from build123d import *

# Parameters (mm, degrees)
ESQUISSE1_W             = 106
ESQUISSE1_H             = 68
BOSS_EXTRU_1_DEPTH      = 8
ESQUISSE2_R             = 3
BOSS_EXTRU_2_DEPTH      = 4.5
ESQUISSE3_R             = 1.25
ENL_V_MAT_EXTRU_1_DEPTH = 7
ESQUISSE4_W             = 106
ESQUISSE4_H             = 1.5
ENL_V_MAT_EXTRU_3_DEPTH = 65
ESQUISSE10_W            = 96
ESQUISSE10_H            = 58.390488624
ENL_V_MAT_EXTRU_5_DEPTH = 1


with BuildPart() as part:
    # Esquisse1 → Boss.-Extru.1 (new body)
    with BuildSketch(Plane(origin=(0, 0, 0), x_dir=(1, 0, 0), z_dir=(0, 1, 0))):
        Rectangle(ESQUISSE1_W, ESQUISSE1_H)
    extrude(amount=BOSS_EXTRU_1_DEPTH)

    # Esquisse2 → Boss.-Extru.2 (add)
    with BuildSketch(Plane.XZ):
        with Locations(Location((-49.5, 31, 0), (0, 0, 90))):
            Circle(ESQUISSE2_R)
        with Locations(Location((-49.5, -31, 0), (0, 0, 90))):
            Circle(ESQUISSE2_R)
        with Locations(Location((49.5, -31, 0), (0, 0, 270))):
            Circle(ESQUISSE2_R)
        with Locations(Location((49.5, 31, 0), (0, 0, 90))):
            Circle(ESQUISSE2_R)
        with Locations(Location((-30.5, 24.5, 0), (0, 0, 90))):
            Circle(ESQUISSE2_R)
        with Locations(Location((27.5, 24.5, 0), (0, 0, 90))):
            Circle(ESQUISSE2_R)
        with Locations(Location((27.5, -24.5, 0), (0, 0, 90))):
            Circle(ESQUISSE2_R)
        with Locations(Location((-30.5, -24.5, 0), (0, 0, 90))):
            Circle(ESQUISSE2_R)
    extrude(amount=BOSS_EXTRU_2_DEPTH)

    # Esquisse3 → Enlèv. mat.-Extru.1 (cut)
    with BuildSketch(Plane.XZ.offset(4.5)):
        with Locations(Location((-49.5, 31, 0), (0, 0, 270))):
            Circle(ESQUISSE3_R)
        with Locations(Location((49.5, 31, 0), (0, 0, 90))):
            Circle(ESQUISSE3_R)
        with Locations(Location((49.5, -31, 0), (0, 0, 270))):
            Circle(ESQUISSE3_R)
        with Locations(Location((-49.5, -31, 0), (0, 0, 90))):
            Circle(ESQUISSE3_R)
        with Locations(Location((-30.5, 24.5, 0), (0, 0, 270))):
            Circle(ESQUISSE3_R)
        with Locations(Location((27.5, 24.5, 0), (0, 0, 90))):
            Circle(ESQUISSE3_R)
        with Locations(Location((27.5, -24.5, 0), (0, 0, 270))):
            Circle(ESQUISSE3_R)
        with Locations(Location((-30.5, -24.5, 0), (0, 0, 90))):
            Circle(ESQUISSE3_R)
    extrude(amount=-ENL_V_MAT_EXTRU_1_DEPTH, mode=Mode.SUBTRACT)

    # Esquisse4 → Enlèv. mat.-Extru.3 (cut)
    with BuildSketch(Plane(origin=(0, 0, -34), x_dir=(-1, 0, 0), z_dir=(0, 0, -1))):
        with Locations((0, 1.75)):
            Rectangle(ESQUISSE4_W, ESQUISSE4_H)
    extrude(amount=-ENL_V_MAT_EXTRU_3_DEPTH, mode=Mode.SUBTRACT)

    # Esquisse10 → Enlèv. mat.-Extru.5 (cut)
    with BuildSketch(Plane(origin=(0, 8, 0), x_dir=(1, 0, 0), z_dir=(0, 1, 0))):
        Rectangle(ESQUISSE10_W, ESQUISSE10_H)
    extrude(amount=-ENL_V_MAT_EXTRU_5_DEPTH, mode=Mode.SUBTRACT)


solid = part.part
Can you work these out from the model? Positions are in its coordinate system, mm. A direction names the side the tool comes from. Coordinates: 2 decimals unless noted, no trailing zeros. Write each loop counter-clockwise with the first axis right and the second up, starting at its lowest first coordinate (ties: lowest second). Pieces come first, ordered by that corner, then holes.
Q1. Imagine slicing it at C-C, the plane z = 11. List the corners of the cut face in (x, y) for me.
Results found:
outline: (-53, 0) - (53, 0) - (53, 1) - (-53, 1) - close; (-53, 2.5) - (53, 2.5) - (53, 8) - (48, 8) - (48, 7) - (-48, 7) - (-48, 8) - (-53, 8) - close
Q2. Please list where these lines run through material, in increasing order: L1, parallel to X at y = -1.25, z = 31; L2, parallel to X at y = -0.3, z = -24.5; L3, parallel to Y at x = 9, z = 9.5.
Results found:
L1: x = -52.5 to -50.75, -48.25 to -46.5, 46.5 to 48.25, 50.75 to 52.5
L2: x = -33.5 to -31.75, -29.25 to -27.5, 24.5 to 26.25, 28.75 to 30.5
L3: y = 0 to 1, 2.5 to 7
Q3. Which directions (+Z, -Z, +X, -X, +Y, -Y) give clear straight access to the entire face, cutting with the end or side of a thin tool? Please do faces 1 (the face through (-30.021, -1.788, -23.345)), 2 (the face through (1, 1, -2)), 3 (the face through (27, -4.5, -23)), 4 (the face through (-1, 7, 0)).
Results found:
face 1: -Y
face 2: -Z, +X, -X
face 3: +Z, -Z, +X, -X, -Y
face 4: +Y
Q4. Imagine slicing it at B-B, the plane z = -24.5. List the corners of the cut face in (x, y) for me.
Results found:
outline: (-53, 0) - (-33.5, 0) - (-33.5, -4.5) - (-31.75, -4.5) - (-31.75, 1) - (-53, 1) - close; (-53, 2.5) - (53, 2.5) - (53, 8) - (48, 8) - (48, 7) - (-48, 7) - (-48, 8) - (-53, 8) - close; (-29.25, -4.5) - (-27.5, -4.5) - (-27.5, 0) - (24.5, 0) - (24.5, -4.5) - (26.25, -4.5) - (26.25, 1) - (-29.25, 1) - close; (28.75, -4.5) - (30.5, -4.5) - (30.5, 0) - (53, 0) - (53, 1) - (28.75, 1) - close
Q5. For P1, Ø4, axis at x = -30.5, z = -24.5, coming from the -Y side; P2, Ø20, axis at x = 15, z = -11, coming from the -Y side; P3, Ø2, axis at x = 49.5, z = -31, coming from the -Y side; P4, Ø19.5, axis at x = -17.5, z = 12.5, coming from the +Y side, each with a flat end and sliding along its axis, tell me the tip position at first contact or that it passes through.
Results found:
P1: stops at y = -4.5
P2: stops at y = 0
P3: stops at y = 2.5
P4: stops at y = 7
Q6. If we mould it in two halves opening along Z, with no side actions, what happens to faces 5 (the face through (27.4, -2.2, -27.5)), 6 (the face through (27, -4.5, 26)), 7 (the face through (-1, 4, 34))? For each: +Z half, -Z half, draft (parallel to the pull), parting line (faces both ways), or undercut.
Results found:
face 5: undercut
face 6: draft
face 7: +Z half
Q7. Imagine slicing it at A-A, the plane x = -30.5. List the corners of the cut face in (y, z) for me.
Results found:
outline: (-4.5, -27.5) - (0, -27.5) - (0, -34) - (1, -34) - (1, -25.75) - (-4.5, -25.75) - close; (-4.5, -23.25) - (1, -23.25) - (1, 23.25) - (-4.5, 23.25) - (-4.5, 21.5) - (0, 21.5) - (0, -21.5) - (-4.5, -21.5) - close; (-4.5, 25.75) - (1, 25.75) - (1, 31) - (2.5, 31) - (2.5, -34) - (8, -34) - (8, -29.2) - (7, -29.2) - (7, 29.2) - (8, 29.2) - (8, 34) - (0, 34) - (0, 27.5) - (-4.5, 27.5) - close
